Study the drawing (mm; zero at the part's minimum x, y, z) and answer. Round coordinates to 2 decimals unless told otherwise and drop trailing zeros. Order: outer loops, then holes, each group sorted by start corner. A loop starts at its lowest first (then second) coordinate and runs counter-clockwise, first axis right, second up. Notation, with made-up numbers: (-15.75, -34.5) - (-1.75, -34.5) arc R37 ccw to (-1.75, 2.5) - close; hole circle Ø3 at (27, -5.5). An arc over 180 degrees is marked (long way). Put each result on its own line as item: value.
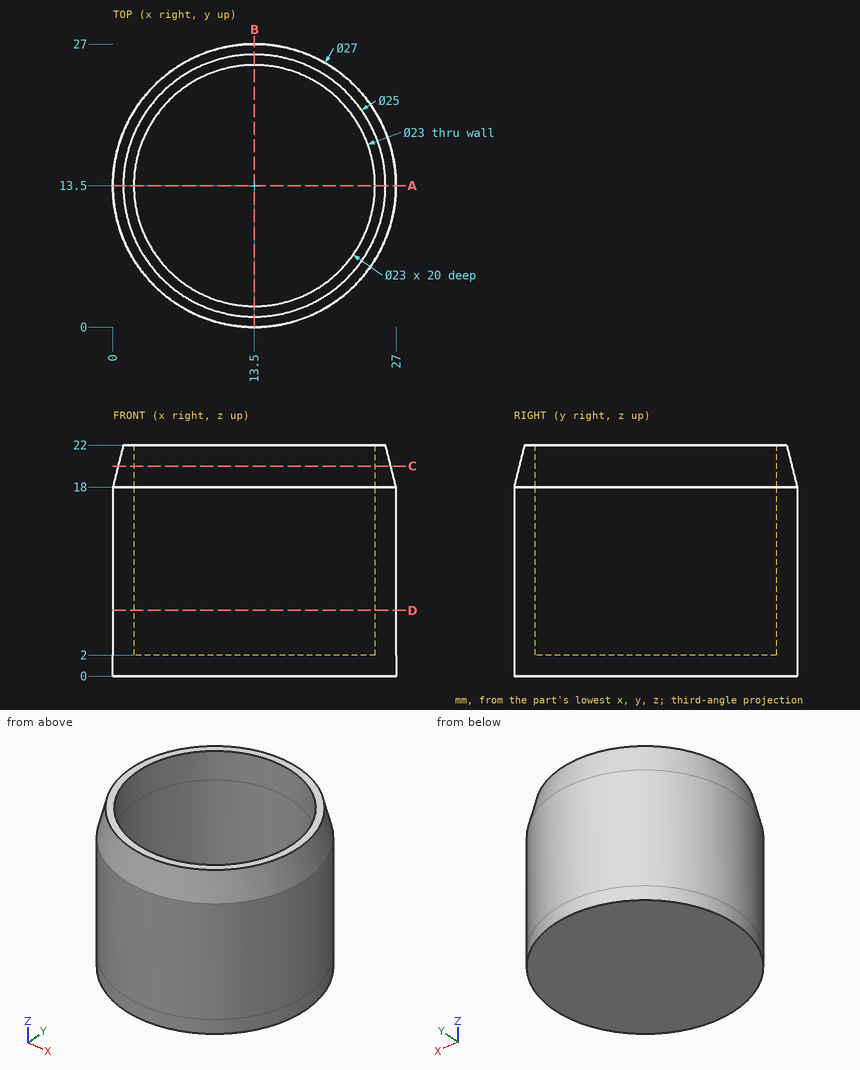
1) A cutting plane is placed at D-D on z = 6.25. Write down the section's boundary in (x, y), then the cut area to 3 significant figures.
Findings below:
outline: circle Ø27 at (13.5, 13.5); hole circle Ø23 at (13.5, 13.5)
area: 157 mm2
2) A cutting plane is placed at C-C on z = 20. Write down the section's boundary in (x, y), then the cut area to 3 significant figures.
Findings below:
outline: circle Ø26 at (13.5, 13.5); hole circle Ø23 at (13.5, 13.5)
area: 115 mm2
3) Straight lines are drawn through the part: L1, parallel to Y at x = 13.5, z = 8; L2, parallel to Z at x = 3.5, y = 11.75; L3, parallel to X at y = 14, z = 14. For each, find the intervals that lie inside material, in ascending order. Write a range as from..to.
Findings below:
L1: y = 0..2, 25..27
L2: z = 0..2
L3: x = 0.01..2.01, 24.99..26.99
4) A cutting plane is placed at A-A on y = 13.5. Write down the section's boundary in (x, z).
Findings below:
outline: (0, 0) - (27, 0) - (27, 18) - (26, 22) - (25, 22) - (25, 2) - (2, 2) - (2, 22) - (1, 22) - (0, 18) - close
5) Given pin 1 Ø4 at (y, z) = (3, 4.5) entering from +X; pin 2 Ø5 at (y, z) = (8.5, 14.5) entering from -X; pin 3 Ø7 at (x, y) = (12, 18.5) entering from +Z, each flat-ended and moving along its own axis, determine where each tip first touches the part or whether it passes through.
Findings below:
pin 1: stops at x = 23.99
pin 2: stops at x = 0.23
pin 3: stops at z = 2
